Could you check a few things on this model? Use its own coordinates, in mm. Face numbers are marked on the shaded views. A direction names the side the tool comes from. Round coordinates to 2 decimals unless told otherwise and drop trailing zeros. Order: outer loops, then holes, each group sorted by start corner. A loop starts at its lowest first (then second) coordinate and runs counter-clockwise, first axis right, second up. Notation, with made-up numbers: M -16,68 L 15,68 A20 cw 15,82 Z; hole C 62,2 d1. An arc over 180 degrees is marked long. Write each question's results on one line, items separated by ' | '. Start each with the question number.
1. Suppose I cut it at D-D on z = -1. Write out the boundary of the cut face in (x, y).
2. Suppose I cut it at C-C on y = 10. Write out the boundary of the cut face in (x, z), and give its area (3 significant figures).
3. We'd pull the mould along X, two halves only. Please class the marked faces 4, 5 and 6: released by +X, released by -X, zero draft, split by the parting line, or undercut.
4. Suppose I cut it at B-B on z = -11. Write out the boundary of the cut face in (x, y).
5. For the marked faces 1, 2 and 3, which set-ups out of +Z, -Z, +X, -X, +Y, -Y let a thin tool reach every point of the face, with its end or its side?
6. I'm going to push flat-ended pins straight in: pin 1 (6 mm diameter, centred on x = 5.5, y = 4.5, fed in from +Z); pin 2 (1.5 mm diameter, centred on x = 6, y = 10, fed in from +Z); pin 3 (4 mm diameter, centred on x = -2, z = -8, fed in from -Y); pin 4 (2.5 mm diameter, centred on y = -6.5, z = -9.5, fed in from +X). Where does each tip first touch, or does it pass through?
7. Suppose I cut it at A-A on x = 6. Write out the boundary of the cut face in (y, z), and give its area (3 significant figures).
8. Please list where these lines run through material, in increasing order: L1, parallel to Y at x = 6, z = -10.8; L2, parallel to Y at x = 6, z = -8.55; L3, parallel to X at y = 4, z = -2.
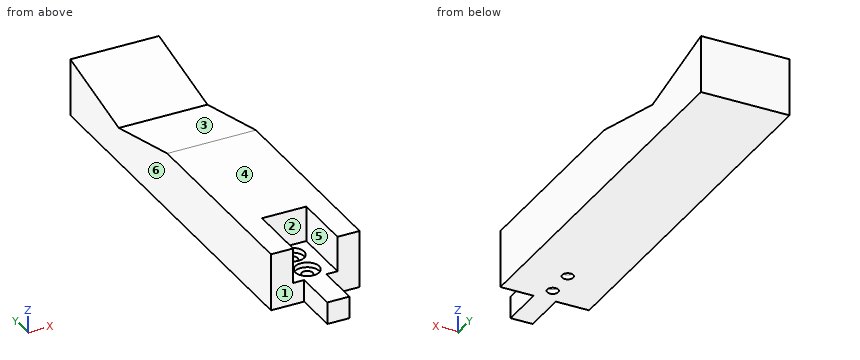
Autodesk Inventor part; units mm, degrees
ref_plane "Work Plane1" through (6, 0, 0) normal (1, 0, 0) x (0, 0, -1)
ref_plane "YZ Plane" through (0, 0, 0) normal (1, 0, 0) x (0, 1, 0)
ref_plane "XZ Plane" through (0, 0, 0) normal (0, 1, 0) x (-1, 0, 0)
sketch "Sketch2" plane through (0, 0, 0) normal (1, 0, 0) x (0, 1, 0)
  line L0 (0, 0) -> (15, 0)
  line L1 (15, 0) -> (15, -10)
  line L2 (15, -10) -> (0, -10)
  line L3 (0, -10) -> (0, 0)
  dimension "d4" = 15
  dimension "d5" = 10
extrude "Extrusion2" add sketch "Sketch2" along normal blind 12
sketch "Sketch3" plane through (0, 0, 0) normal (0, 0, 1) x (1, 0, 0)
  line L0 (0, 0) -> (1, 0)
  line L1 (0, 0) -> (12, 0)
  line L2 (1, 0) -> (1, 13.5)
  line L3 (1, 13.5) -> (11, 13.5)
  line L4 (11, 13.5) -> (11, 0)
  line L5 (11, 0) -> (1, 0)
  dimension "d8" = 1
  dimension "d9" = 13.5
  dimension "d10" = 10
extrude "Extrusion3" cut sketch "Sketch3" against normal blind 8
sketch "Sketch4" plane through (0, 0, -10) normal (0, 0, -1) x (-1, 0, 0)
  line L0 (0, 15) -> (-12, 15)
  line L1 (0, 0) -> (-12, 0)
  line L2 (-12, 15) -> (0, 15)
  line L3 (0, 15) -> (0, 0)
  line L4 (0, 0) -> (-12, 0)
  line L5 (-12, 0) -> (-12, 15)
extrude "Extrusion4" add sketch "Sketch4" along normal blind 2
sketch "Sketch5" plane through (0, 0, -8) normal (0, 0, 1) x (1, 0, 0)
  line L0 (1, 13.5) -> (11, 13.5)
  line L1 (6, 13.5) -> (6, 10)
  line L2 (6, 10) -> (6, 3.5)
  circle A0 centre (6, 10) radius 1.2295
  circle A1 centre (6, 3.5) radius 1.2295
  point P0 (0, 0)
  dimension "d15" = 3.5
  dimension "d16" = 6.5
  dimension "d17" = 2.459
  dimension "d18" = 2.459
extrude "Extrusion5" cut sketch "Sketch5" against normal blind 4
sketch "Sketch6" plane through (0, 0, -8) normal (0, 0, 1) x (1, 0, 0)
  circle A0 centre (6, 10) radius 1.2295
  circle A1 centre (6, 10) radius 2.7
  circle A2 centre (6, 3.5) radius 1.2295
  circle A3 centre (6, 3.5) radius 2.7
  point P0 (0, 0)
  dimension "d21" = 5.4
  dimension "d22" = 5.4
extrude "Extrusion6" cut sketch "Sketch6" against normal blind 1.1
sketch "Sketch15" plane through (12, 0, 0) normal (1, 0, 0) x (0, 0, -1)
  line L0 (0, 15) -> (12, 15)
  line L1 (12, 15) -> (12, 0)
  line L2 (0, 15) -> (12, 15)
  line L3 (12, 15) -> (12, 0)
  line L4 (12, 0) -> (0, 0)
  line L5 (0, 0) -> (0, 15)
extrude "Extrusion14" add sketch "Sketch15" along normal blind 4
ref_plane "Work Plane1" through (6, 0, 0) normal (1, 0, 0) x (0, 0, -1)
mirror "Mirror1" about plane through (6, 0, 0) normal (1, 0, 0) of "Extrusion14"
sketch "Sketch16" plane through (1, 0, -8) normal (0, -1, 0) x (1, 0, 0)
  line L0 (10, 0) -> (0, 0)
  line L1 (5, 0) -> (7.5, 0)
  line L2 (7.5, 0) -> (7.5, -4)
  line L3 (-5, -4) -> (15, -4)
  line L4 (7.5, -4) -> (2.5, -4)
  line L5 (2.5, -4) -> (2.5, 0)
  line L6 (2.5, 0) -> (5, 0)
  point P0 (-1, 8)
  dimension "d61" = 2.5
  dimension "d62" = 4
  dimension "d63" = 5
  dimension "d64" = 4
extrude "Extrusion15" add sketch "Sketch16" along normal blind 10
sketch "Sketch18" plane through (0, 0, -12) normal (0, 0, -1) x (-1, 0, 0)
  line L0 (-16, 15) -> (4, 15)
  line L1 (4, 0) -> (-3.5, 0)
  line L2 (-16, 15) -> (4, 15)
  line L3 (4, 15) -> (4, 0)
  line L4 (4, 0) -> (-16, 0)
  line L5 (-16, 0) -> (-16, 15)
  line L6 (-8.5, -10) -> (-3.5, -10)
  line L7 (-3.5, 0) -> (-8.5, 0)
  line L8 (-8.5, 0) -> (-8.5, -10)
  line L9 (-8.5, -10) -> (-3.5, -10)
  line L10 (-3.5, -10) -> (-3.5, 0)
  circle A0 centre (-6, 3.5) radius 1.2295
  circle A1 centre (-6, 3.5) radius 1.2295
  circle A2 centre (-6, 10) radius 1.2295
  circle A3 centre (-6, 10) radius 1.2295
  point P0 (0, 0)
extrude "Extrusion16" add sketch "Sketch18" along normal blind 1
sketch "Sketch19" plane through (16, 0, 0) normal (1, 0, 0) x (0, 0, -1)
  line L0 (0, 15) -> (13, 15)
  line L1 (0, 15) -> (0, 40)
  line L2 (13, 45) -> (13, 15)
  line L3 (13, 56) -> (13, 45)
  line L4 (0, 45) -> (0, 40)
  line L5 (13, 60) -> (13, 56)
  line L6 (13, 61) -> (13, 60)
  line L7 (0, 87) -> (13, 87)
  line L8 (13, 87) -> (13, 61)
  line L9 (5, 66) -> (0, 87)
  line L10 (5, 66) -> (0, 45)
  point P0 (0, 0)
extrude "Extrusion17" add sketch "Sketch19" against normal blind 20
properties part number "40mm_x_20mm"
Filled sheet:
1) outline: M -4,0 L 1,0 L 1,13.5 L 11,13.5 L 11,0 L 16,0 L 16,49.2 L -4,49.2 Z; M -4,82.8 L 16,82.8 L 16,87 L -4,87 Z
2) outline: M -4,-13 L 4.77,-13 L 4.77,-9.1 L 3.3,-9.1 L 3.3,-8 L 1,-8 L 1,0 L -4,0 Z; M 7.23,-13 L 16,-13 L 16,0 L 11,0 L 11,-8 L 8.7,-8 L 8.7,-9.1 L 7.23,-9.1 Z | area: 164 mm^2
3) face 4: zero draft | face 5: undercut | face 6: released by -X
4) outline: M -4,0 L 3.5,0 L 3.5,-10 L 8.5,-10 L 8.5,0 L 16,0 L 16,87 L -4,87 Z; hole C 6,3.5 d2.46; hole C 6,10 d2.46
5) face 1: +Z, -Z, -X, -Y | face 2: +Z, -Y | face 3: +Z, +X, -X
6) pin 1: stops at z = -8 | pin 2: passes through | pin 3: stops at y = 0 | pin 4: stops at x = 8.5
7) outline: M -10,-13 L 2.27,-13 L 2.27,-9.1 L 0.8,-9.1 L 0.8,-8 L -10,-8 Z; M 4.73,-13 L 8.77,-13 L 8.77,-9.1 L 7.3,-9.1 L 7.3,-8 L 6.2,-8 L 6.2,-9.1 L 4.73,-9.1 Z; M 11.23,-13 L 87,-13 L 87,0 L 66,-5 L 45,0 L 13.5,0 L 13.5,-8 L 12.7,-8 L 12.7,-9.1 L 11.23,-9.1 Z | area: 937 mm^2
8) L1: y = -10 to 2.27, 4.73 to 8.77, 11.23 to 87 | L2: y = -10 to 0.8, 6.2 to 7.3, 12.7 to 87 | L3: x = -4 to 1, 11 to 16
